The listing builds one solid part. Answer for the finished solid, in the listing's coordinates (mm). A direction names the side the tool comes from. Coordinates: 2 decimals unless noted, no trailing zeros. Loops run counter-clockwise (first coordinate to the right, second up) from the corner with the lowest first, then second, coordinate; pieces in that order, holes last. Notation, with made-up numbers: (-14, 33.5) - (30, 33.5) arc R17 ccw to (30, 37.5) - close; hole circle Ø11 at (-17, 45). An arc over 180 degrees is marked (long way). Write each question's results on one line, items separated by ' | '. Start each with the question number.
(1) Determine the mould class of faces 4 (the flat face through (6.89, 0.05, 0)), 5 (the flat face through (4.542, 2.254, 7.888)) for opening direction X: released by +X, released by -X, zero draft, split by the parting line, or undercut.
(2) Find section D-D on y = -1. Determine the outline of the cut face in (x, z).
(3) For faces 1 (the flat face through (4.69, -1.2, 7.89)), 2 (the flat face through (9.22, 2.246, 7.888)), 3 (the cylindrical face through (-3.246, -0.153, 7.888)), determine the directions among +Z, -Z, +X, -X, +Y, -Y from which every point of the face is accessible in a straight line to the end or side of a thin tool.
(4) Find section C-C on y = 1. Determine the outline of the cut face in (x, z).
(5) Consider line 1 (Y direction, x = 0, z = 5.5); line 2 (Y direction, x = 1.5, z = 1); line 3 (X direction, y = -2.75, z = 3.25). Determine where each line is inside the solid, lowest interval first. Write a range as from..to.
(6) Given pin 1 Ø2 at (y, z) = (1.5, 5.5) entering from -X; pin 2 Ø1 at (x, z) = (1, 2.5) entering from -Y, each flat-ended and moving along its own axis, determine where each tip first touches the part or whether it passes through.
(7) Find section A-A on z = 5.5. Determine the outline of the cut face in (x, y).
(8) Find section B-B on x = 0. Determine the outline of the cut face in (y, z).
from build123d import *

# Parameters (mm, degrees)
SKETCH1_R           = 2
BOSS_EXTRUDE1_DEPTH = 16


with BuildPart() as part:
    # Sketch1 → Boss-Extrude1 (new body)
    with BuildSketch(Plane.XY):
        with BuildLine():
            Line((2.076655966, 2.5), (7.076655966, 2))
            Line((7.076655966, 2), (11.423344034, 2.5))
            ThreePointArc((11.423344034, 2.5), (16.75, 0), (11.423344034, -2.5))
            Line((11.423344034, -2.5), (7.151636088, 0))
            Line((7.151636088, 0), (2.151636088, -2.43576726))
            ThreePointArc((2.151636088, -2.43576726), (-3.249625061, -0.049365635), (2.076655966, 2.5))
        make_face()
        Circle(SKETCH1_R, mode=Mode.SUBTRACT)
    extrude(amount=BOSS_EXTRUDE1_DEPTH)


solid = part.part
Values:
1) face 4: zero draft | face 5: undercut
2) outline: (-3.09, 0) - (-1.73, 0) - (-1.73, 16) - (-3.09, 16) - close; (1.73, 0) - (5.1, 0) - (5.1, 16) - (1.73, 16) - close; (8.86, 0) - (16.59, 0) - (16.59, 16) - (8.86, 16) - close
3) face 1: +Z, -Z, -Y | face 2: +Z, -Z, +Y | face 3: +Z, -Z
4) outline: (-3.09, 0) - (-1.73, 0) - (-1.73, 16) - (-3.09, 16) - close; (1.73, 0) - (16.59, 0) - (16.59, 16) - (1.73, 16) - close
5) line 1: y = -3.25..-2, 2..3.25 | line 2: y = -2.88..-1.32, 1.32..2.88 | line 3: x = -1.73..1.73, 11.77..15.23
6) pin 1: stops at x = -3.21 | pin 2: stops at y = -3.21
7) outline: (2.08, 2.5) arc R3.25 ccw (long way) to (2.15, -2.44) - (7.15, 0) - (11.42, -2.5) arc R3.25 ccw (long way) to (11.42, 2.5) - (7.08, 2) - close; hole circle Ø4 at (0, 0)
8) outline: (-3.25, 0) - (-2, 0) - (-2, 16) - (-3.25, 16) - close; (2, 0) - (3.25, 0) - (3.25, 16) - (2, 16) - close
